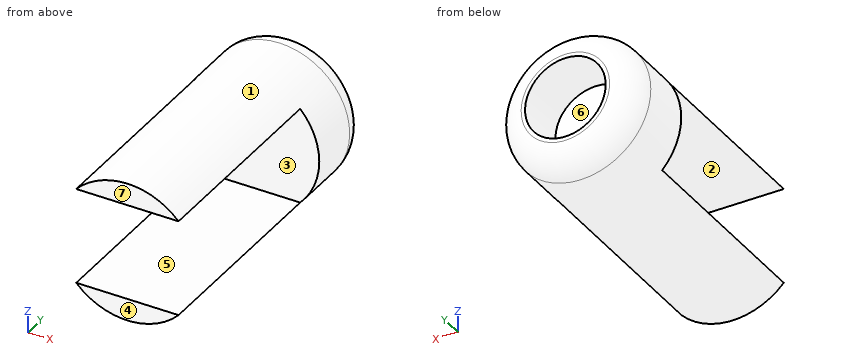
```python
from build123d import *

# Parameters (mm, degrees)
SKETCH1_R           = 2.7
BOSS_EXTRUDE1_DEPTH = 11
CUT_EXTRUDE1_DEPTH  = 8
SKETCH3_R           = 1.55
CUT_EXTRUDE2_DEPTH  = 2
FILLET1_R           = 1


with BuildPart() as part:
    # Sketch1 → Boss-Extrude1 (new body)
    with BuildSketch(Plane(origin=(0, 0, 0), x_dir=(1, 0, 0), z_dir=(0, 1, 0))):
        with Locations(Location((0, 0, 0), (0, 0, 270))):
            Circle(SKETCH1_R)
    extrude(amount=BOSS_EXTRUDE1_DEPTH)

    # Sketch2 → Cut-Extrude1 (cut)
    with BuildSketch(Plane.XZ):
        with BuildLine():
            Line((1.966596044, 1.85), (-1.966596044, 1.85))
            ThreePointArc((-1.966596044, 1.85), (-2.7, 0), (-1.966596044, -1.85))
            Line((-1.966596044, -1.85), (1.966596044, -1.85))
            ThreePointArc((1.966596044, -1.85), (2.7, 0), (1.966596044, 1.85))
        make_face()
    extrude(amount=-CUT_EXTRUDE1_DEPTH, mode=Mode.SUBTRACT)

    # Sketch3 → Cut-Extrude2 (cut)
    with BuildSketch(Plane(origin=(0, 11, 0), x_dir=(1, 0, 0), z_dir=(0, 1, 0))):
        with Locations(Location((0, 0, 0), (0, 0, 270))):
            Circle(SKETCH3_R)
    extrude(amount=-CUT_EXTRUDE2_DEPTH, mode=Mode.SUBTRACT)

    # Fillet1
    fillet1_edges = [part.edges().sort_by_distance(p)[0] for p in [
        (0, 11, -2.7),
    ]]
    fillet(fillet1_edges, radius=FILLET1_R)


solid = part.part
```
Verification items for the finished model (mm, model axes). Face numbers are marked on the shaded views. A direction names the side the tool comes from. Round coordinates to 2 decimals unless told otherwise and drop trailing zeros. Order: outer loops, then holes, each group sorted by start corner. A loop starts at its lowest first (then second) coordinate and runs counter-clockwise, first axis right, second up. Notation, with made-up numbers: (-5.75, 44) -> (44.25, 44) arc R17 cw to (44.25, 62) -> close; hole circle Ø6 at (87.5, 85.25). An arc over 180 degrees is marked (long way). Put each result on its own line as item: value. Start each with the question number.
(1) Section check C-C (y = 6.5). Enter the section's corners in (x, z), then the cut area to 3 significant figures.
(2) Section check A-A (x = 0). Enter the section's corners in (y, z), then the cut area to 3 significant figures.
(3) Section check D-D (y = 8.75). Enter the section's corners in (x, z).
(4) Draft check along Z on the marked faces 1, 2, 3 and 4. Enter one of: +Z half, -Z half, draft (parallel to the pull), parting line (faces both ways), or undercut.
(5) Tool access check on the marked faces 5, 6 and 7. Record the directions out of +Z, -Z, +X, -X, +Y, -Y that give a thin tool (end or side, any length) a straight path to the whole face; none if there is none.
(6) Depth check by flat-ended pin: pin 1 Ø1.5 at (y, z) = (2, 0.5) entering from +X; pin 2 Ø2.5 at (x, z) = (0, 0) entering from -Y; pin 3 Ø0.9 at (x, z) = (-0.5, 0) entering from +Y; pin 4 Ø2 at (x, y) = (1.5, 3) entering from +Z. Enter the tip coordinate at first touch or a pass-through.
(7) Section check B-B (z = 0). Enter the section's corners in (x, y).
(8) Material ranges on line 1 along X through (y, z) = (9.65, 0); line 2 along Y through (x, z) = (-1.6, 0.55); line 3 along Y through (x, z) = (0.1, -1.25), recorded low to high.
Completed:
1. outline: (-1.97, -1.85) arc R2.7 ccw to (1.97, -1.85) -> close; (-1.97, 1.85) -> (1.97, 1.85) arc R2.7 ccw to start
1. area: 4.62 mm2
2. outline: (0, -2.7) -> (10, -2.7) arc R1 ccw to (11, -1.7) -> (11, -1.55) -> (9, -1.55) -> (9, 1.55) -> (11, 1.55) -> (11, 1.7) arc R1 ccw to (10, 2.7) -> (0, 2.7) -> (0, 1.85) -> (8, 1.85) -> (8, -1.85) -> (0, -1.85) -> close
2. area: 23.2 mm2
3. outline: circle Ø5.4 at (0, 0)
4. face 1: parting line
4. face 2: undercut
4. face 3: undercut
4. face 4: draft
5. face 5: +X, -X, -Y
5. face 6: +Y
5. face 7: +Z, -Z, +X, -X, -Y
6. pin 1: passes through
6. pin 2: stops at y = 8
6. pin 3: stops at y = 9
6. pin 4: stops at z = 2.65
7. outline: (-2.7, 8) -> (2.7, 8) -> (2.7, 10) arc R1 ccw to (1.7, 11) -> (1.55, 11) -> (1.55, 9) -> (-1.55, 9) -> (-1.55, 11) -> (-1.7, 11) arc R1 ccw to (-2.7, 10) -> close
8. line 1: x = -2.7 to -1.55, 1.55 to 2.7
8. line 2: y = 8 to 11
8. line 3: y = 8 to 9
